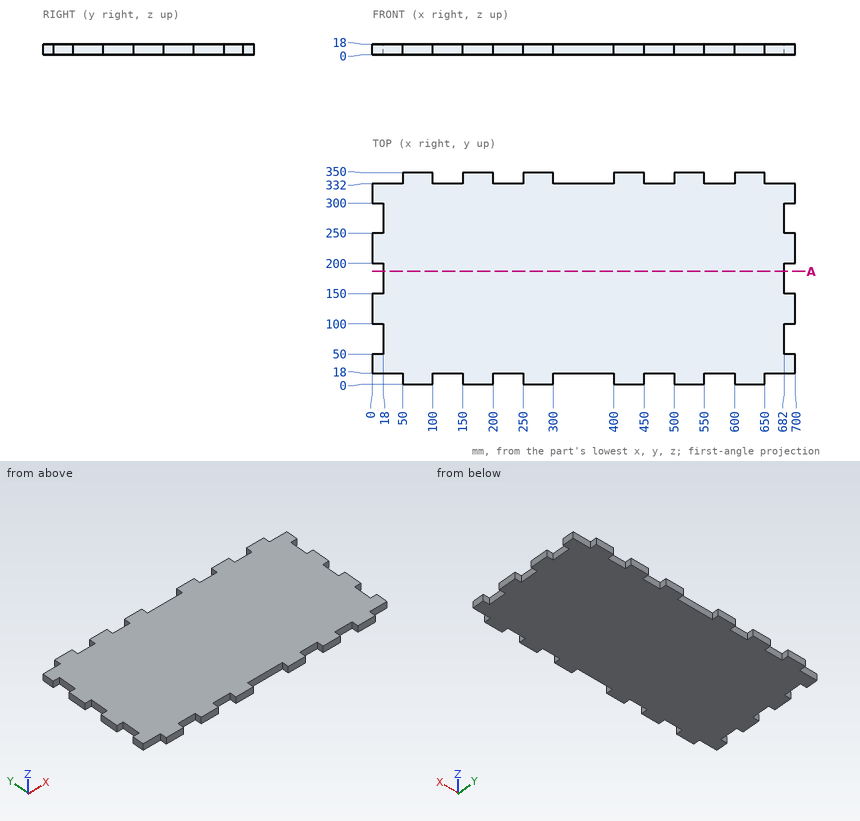
For this review, use the dimensioned drawing (mm, ordinates from the lowest corner) and the shaded views. Round coordinates to 2 decimals unless told otherwise and drop trailing zeros. Order: outer loops, then holes, each group sorted by start corner. A loop starts at its lowest first (then second) coordinate and runs counter-clockwise, first axis right, second up. Notation, with made-up numbers: (-1, 86.5) -> (40, 86.5) arc R20 cw to (40, 95.5) -> close; hole circle Ø3 at (-16.75, -33.5). An arc over 180 degrees is marked (long way). One line per item, written item: value. Start each with the question number.
Q1. Clearance check with flat-ended pins moving along their axes: pin 1 Ø3 at (x, z) = (597.5, 2.5) entering from -Y; pin 2 Ø5.5 at (x, z) = (465, 9.5) entering from +Y; pin 3 Ø9 at (y, z) = (6.5, 6) entering from -X; pin 4 Ø5 at (x, z) = (622.5, 3.5) entering from -Y. State where each tip first meets the part, or that it passes through.
Q2. Wall thickness on line 1 (X direction, y = 162, z = 15.5); line 2 (Y direction, x = 373.5, z = 7.75): over which ranges is each line inside the solid? List them lowest first.
Q3. Take a section at A-A (y = 187). Write out the cut boundary in (x, z), and give its area (3 significant figures).
Reported:
1. pin 1: stops at y = 18
1. pin 2: stops at y = 332
1. pin 3: stops at x = 50
1. pin 4: stops at y = 0
2. line 1: x = 18 to 682
2. line 2: y = 18 to 332
3. outline: (18, 0) -> (682, 0) -> (682, 18) -> (18, 18) -> close
3. area: 12,000 mm2
